Verification items for the finished model (mm, model axes). Round coordinates to 2 decimals unless told otherwise and drop trailing zeros. Write each loop counter-clockwise with the first axis right and the second up, starting at its lowest first coordinate (ties: lowest second). Pieces come first, ordered by that corner, then holes. Notation, with made-up numbers: M 76,3 L 101,3 A15 cw 101,10 Z; hole C -31,-18 d3. An arc over 180 degrees is marked long. One line per item, written item: value. Start each with the question number.
Item 1: Section check A-A, the plane x = 0. Record the cut outline in (y, z).
Item 2: Section check C-C, the plane y = -18. Record the cut outline in (x, z).
Item 3: Thickness scan on probe 1 along Y at (x, z) = (0, 0.5); probe 2 along Y at (x, z) = (0, 4.5); probe 3 along X at (y, z) = (-4.5, -2.5). Record the ranges inside material, lowest first. Write a range as from..to.
Item 4: Section check B-B, the plane z = 57. Record the cut outline in (x, y), then the cut area to 3 significant figures.
Item 5: Draft check along Y on faces 1 (the face through (-6.466, 2.681, 0.542)), 2 (the face through (-7, -3, 15)). Enter one of: +Y half, -Y half, draft (parallel to the pull), parting line (faces both ways), or undercut.
Item 6: Gauge pin test, flat ends, axial feed: pin 1 (14.5 mm diameter, centred on x = 0.5, y = -5.5, fed in from +Z); pin 2 (3 mm diameter, centred on x = 6, z = 0, fed in from -Y); pin 3 (10 mm diameter, centred on x = 80.5, y = -0.5, fed in from +Z); pin 4 (12 mm diameter, centred on x = 100, y = 16, fed in from -Z). Record the tip position at first contact, or that the pin passes through.
from build123d import *

# Parameters (mm, degrees)
F3_T4_ANGLE = 342.0779351193
F5_D        = 14


# Not quite as in the source:
# - a fillet or chamfer that OpenCascade refuses, or shapes differently, is made with other operations: its cross-section is extruded or revolved along the edge and cut away or added


with BuildPart() as f1:
    # F0 (on Front) → F1 (revolve)
    with BuildSketch(Plane.XZ):
        with BuildLine():
            Line((0, 15), (-14.6969384567, 15))
            ThreePointArc((-14.6969384567, 15), (-21, 0), (-14.6969384567, -15))
            Line((-14.6969384567, -15), (0, -15))
            Line((0, -15), (0, -14.1738577821))
            Line((0, -14.1738577821), (0, 0))
            Line((0, 0), (0, 13.5706276966))
            Line((0, 13.5706276966), (0, 15))
        make_face()
    revolve(axis=Axis((0, 0, 0), (0, 0, -1)))

    # F0 (on Front) → F2 (revolve)
    with BuildSketch(Plane.XZ):
        with BuildLine():
            Line((116.5621770938, 48.278140652), (12.0901276659, 17.1705798686))
            Line((12.0901276659, 17.1705798686), (4.800423118, 15))
            Line((4.800423118, 15), (0, 13.5706276966))
            Line((0, 13.5706276966), (0, 0))
            Line((0, 0), (19.7335450365, 7.1824230098))
            Line((19.7335450365, 7.1824230098), (117.4615775982, 42.7525179157))
            ThreePointArc((117.4615775982, 42.7525179157), (116.7518070973, 45.4729978899), (116.5621770938, 48.278140652))
        make_face()
        with BuildLine():
            ThreePointArc((145.6523562218, 53.0131222155), (129.1471447343, 62.6879798784), (116.5621770938, 48.278140652))
            ThreePointArc((116.5621770938, 48.278140652), (116.7518070973, 45.4729978899), (117.4615775982, 42.7525179157))
            Line((117.4615775982, 42.7525179157), (145.6523562218, 53.0131222155))
        make_face()
    revolve(axis=Axis((72.8261781109, 0, 26.5065611077), (0.9396926208, 0, 0.3420201433)))

    # F3: fillet of radius 5 on 2 edges, made by hand


with BuildPart() as f3_tool2:
    # F3_s3 → F3_t4 (revolve)
    with BuildSketch(Plane(origin=(1e-10, -2.3e-09, -3e-10), x_dir=(-0.9985488213, -0.053853982, 0), z_dir=(-0.0532739776, 0.9877945051, 0.1463690505))):
        with BuildLine():
            ThreePointArc((-10.2959142188, 18.3028453824), (-12.2007985149, 17.6906243055), (-14.1932009283, 17.8742855481))
            Line((-14.1932009283, 17.8742855481), (-12.0219430441, 17.2183880011))
            ThreePointArc((-12.0219430441, 17.2183880011), (-11.1720947014, 17.7815718865), (-10.2959142188, 18.3028453824))
        make_face()
    revolve(axis=Axis((16.194369394, 1.4e-09, 5.8942683966), (0.9396926208, 0, 0.3420201433)), revolution_arc=F3_T4_ANGLE)

    split(bisect_by=Plane.XY.offset(15), keep=Keep.BOTTOM)


with BuildPart() as f1_1:
    add(f1.part)

    # F3_t1: union F3_tool2
    add(f3_tool2.part)

    # F3_s6 → F3_t7 (revolve)
    with BuildSketch(Plane.XZ):
        with BuildLine():
            ThreePointArc((113.4424776902, 47.3492200522), (115.6809078185, 48.7404946697), (116.9009348123, 51.0766771615))
            ThreePointArc((116.9009348123, 51.0766771615), (116.6656687231, 49.6853844353), (116.5621770938, 48.278140652))
            Line((116.5621770938, 48.278140652), (113.4424776902, 47.3492200522))
        make_face()
    revolve(axis=Axis((118.4432878821, 0, 43.1098312377), (0.9396926208, 0, 0.3420201433)))

    # F5 (through all)
    with Locations(Plane(origin=(0, 0, -15), x_dir=(1, 0, 0), z_dir=(0, 0, -1))):
        with Locations((0, 0)):
            Hole(F5_D / 2)


solid = f1_1.part
Response values:
1. outline: M -14.7,-15 L -7,-15 L -7,15 L -14.7,15 A21 ccw Z; M 7,-15 L 14.7,-15 A21 ccw 14.7,15 L 7,15 Z
2. outline: C 0,0 d21.63
3. probe 1: y = -20.99..-7, 7..20.99
3. probe 2: y = -20.51..-7, 7..20.51
3. probe 3: x = -20.36..-5.36, 5.36..24.69
4. outline: C 131.56,0 d23.82
4. area: 446 mm2
5. face 1: undercut
5. face 2: draft
6. pin 1: stops at z = 15.44
6. pin 2: stops at y = -20.51
6. pin 3: stops at z = 39.02
6. pin 4: passes through
